from build123d import *

# Parameters (mm, degrees)
CROQUIS1_R              = 1.6
SALIENTE_EXTRUIR1_DEPTH = 2.6
CROQUIS3_W              = 1
CROQUIS3_H              = 15.5
SALIENTE_EXTRUIR2_DEPTH = 2.6
CORTAR_EXTRUIR1_DEPTH   = 35.458997374
REDONDEO1_R             = 3


with BuildPart() as part:
    # Croquis1 → Saliente-Extruir1 (new body)
    with BuildSketch(Plane(origin=(0, 0, 0), x_dir=(1, 0, 0), z_dir=(0, 1, 0))):
        with BuildLine():
            Line((-3.25, 30.9), (-3.25, 0))
            ThreePointArc((-3.25, 0), (-2.298097039, -2.298097039), (0, -3.25))
            Line((0, -3.25), (2.8, -3.25))
            Line((2.8, -3.25), (2.8, 34.15))
            Line((2.8, 34.15), (0, 34.15))
            ThreePointArc((0, 34.15), (-2.298097039, 33.198097039), (-3.25, 30.9))
        make_face()
        with Locations(Location((0, 0, 0), (0, 0, 270))):
            Circle(CROQUIS1_R, mode=Mode.SUBTRACT)
        with Locations(Location((0, 30.9, 0), (0, 0, 270))):
            Circle(CROQUIS1_R, mode=Mode.SUBTRACT)
    extrude(amount=SALIENTE_EXTRUIR1_DEPTH)

    # Croquis3 → Saliente-Extruir2 (add)
    with BuildSketch(Plane(origin=(0, 2.6, 0), x_dir=(1, 0, 0), z_dir=(0, 1, 0))):
        with Locations((3.3, 15.45)):
            Rectangle(CROQUIS3_W, CROQUIS3_H)
    extrude(amount=-SALIENTE_EXTRUIR2_DEPTH)

    # Croquis2 → Cortar-Extruir1 (cut, through all)
    with BuildSketch(Plane(origin=(0, 2.6, 0), x_dir=(1, 0, 0), z_dir=(0, 1, 0))):
        with BuildLine():
            Line((-2, 20.2), (-3.25, 20.2))
            Line((-3.25, 20.2), (-3.25, 10.7))
            Line((-3.25, 10.7), (-2, 10.7))
            ThreePointArc((-2, 10.7), (2.75, 15.45), (-2, 20.2))
        make_face()
    extrude(amount=-CORTAR_EXTRUIR1_DEPTH, mode=Mode.SUBTRACT)

    # Redondeo1
    redondeo1_edges = [part.edges().sort_by_distance(p)[0] for p in [
        (-3.25, 1.3, -10.7),
        (-3.25, 1.3, -20.2),
    ]]
    fillet(redondeo1_edges, radius=REDONDEO1_R)


solid = part.part
Model file for the job. Use its own axes, mm. A direction names the side the tool comes from. Round coordinates to 2 decimals unless told otherwise and drop trailing zeros. Loops run counter-clockwise (first coordinate to the right, second up) from the corner with the lowest first, then second, coordinate; pieces in that order, holes last. Notation, with made-up numbers: M 0,88 L 56,88 A30 cw 56,114 Z; hole C -36,58 d1. An arc over 180 degrees is marked long. One line per question, with ' | ' between items.
1) Drill centre lines: line 1 along Z through (x, y) = (-0.75, 0.6); line 2 along X through (y, z) = (0.3, 0); line 3 along Z through (x, y) = (0.5, 0.7). Where is each one in solid material? Low to high.
Solved:
line 1: z = -34.06 to -32.31, -29.49 to -20.03, -10.87 to -1.41, 1.41 to 3.16 | line 2: x = -3.25 to -1.6, 1.6 to 2.8 | line 3: z = -34.15 to -32.42, -29.38 to -19.49, -11.41 to -1.52, 1.52 to 3.25
2) 3-axis set-ups, long thin cutter, end or side, ignore diameter. For faces 4 (the flat face through (3, 1, -7.7)), 5 (the flat face through (3, 1, -23.2)), 6 (the flat face through (3, 0, -16)): which of +Z, -Z, +X, -X, +Y, -Y reach the whole face in a straight line?
Solved:
face 4: +Z, +X, +Y, -Y | face 5: -Z, +X, +Y, -Y | face 6: +Z, -Z, +X, -X, -Y
3) Mould opens along Z. For faces 1 (the flat face through (3, 2.6, -16)), 2 (the cylindrical face through (2.75, 1.32, -15.36)), 3 (the cylindrical face through (-2.323, 1.282, 2.273)) say: +Z half, -Z half, draft (parallel to the pull), parting line (faces both ways), or undercut.
Solved:
face 1: draft | face 2: undercut | face 3: +Z half
4) Flat gauge pins, fed straight in: pin 1 (1.9 mm diameter, centred on x = 0, z = -30.9, fed in from -Y); pin 2 (0.8 mm diameter, centred on x = 3.5, y = 1, fed in from -Z); pin 3 (1.1 mm diameter, centred on x = 3.5, y = 1, fed in from +Z). Where does each tip first touch, or does it go through?
Solved:
pin 1: passes through | pin 2: stops at z = -23.2 | pin 3: stops at z = -7.7
5) Band-saw the part on C-C (y = 0.55). Give the number of separate pieces and of enclosed holes in the cut face, then the cut area to 3 significant figures.
Solved:
separate pieces: 1 | enclosed holes: 2 | area: 171 mm²
6) Band-saw the part on D-D (x = 2). Give the cut face in (y, z), then the cut area to 3 significant figures.
Solved:
outline: M 0,-34.15 L 2.6,-34.15 L 2.6,-18.01 L 0,-18.01 Z; M 0,-12.89 L 2.6,-12.89 L 2.6,3.25 L 0,3.25 Z | area: 83.9 mm²
7) Band-saw the part on B-B (z = 0.5). Give the cut face in (x, y).
Solved:
outline: M -3.21,0 L -1.52,0 L -1.52,2.6 L -3.21,2.6 Z; M 1.52,0 L 2.8,0 L 2.8,2.6 L 1.52,2.6 Z
8) Band-saw the part on A-A (x = -0.5). Give the cut face in (y, z).
Solved:
outline: M 0,-34.11 L 2.6,-34.11 L 2.6,-32.42 L 0,-32.42 Z; M 0,-29.38 L 2.6,-29.38 L 2.6,-19.96 L 0,-19.96 Z; M 0,-10.94 L 2.6,-10.94 L 2.6,-1.52 L 0,-1.52 Z; M 0,1.52 L 2.6,1.52 L 2.6,3.21 L 0,3.21 Z
